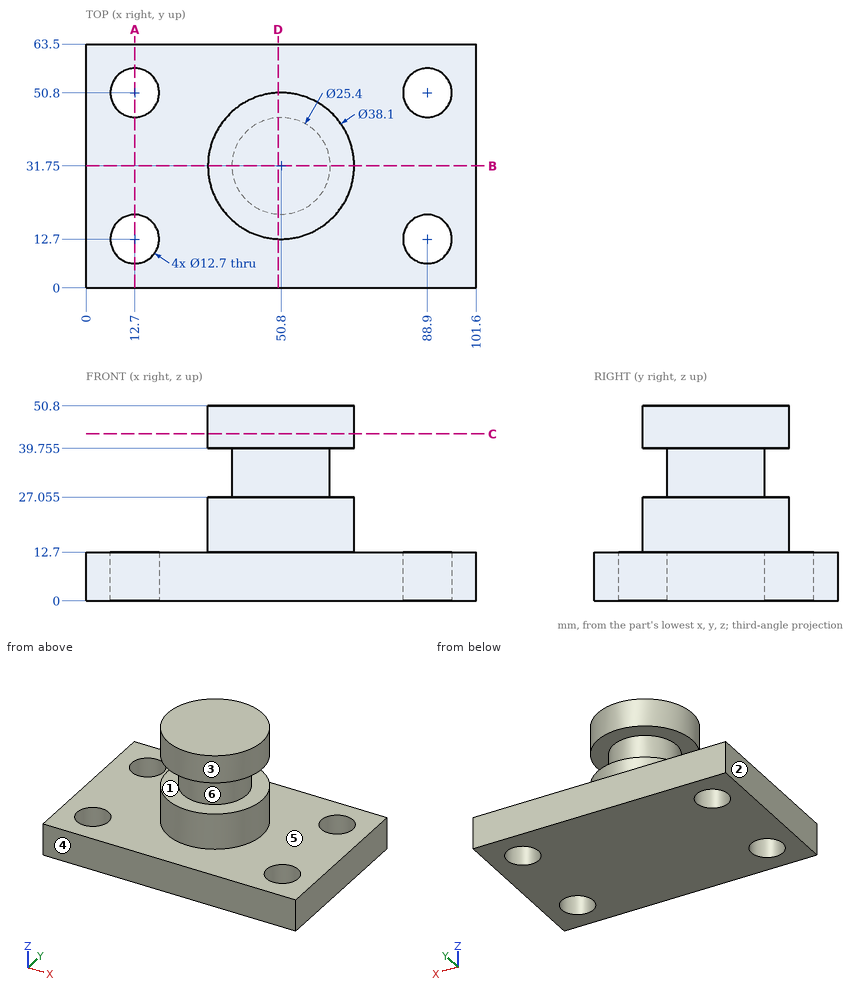
For this review, use the dimensioned drawing (mm, ordinates from the lowest corner) and the shaded views. A direction names the side the tool comes from. Coordinates: 2 decimals unless noted, no trailing zeros. Write each loop counter-clockwise with the first axis right and the second up, starting at its lowest first coordinate (ties: lowest second). Pieces come first, ordered by that corner, then holes. Notation, with made-up numbers: (65, 43) -> (83, 43) arc R25 cw to (83, 80) -> close; hole circle Ø2 at (28.5, 8). An arc over 180 degrees is marked (long way). Put each result on its own line as item: value.
Q1. Take a section at A-A, the plane x = 12.7. State the section outline as (y, z) points, then the cut area to 3 significant figures.
From the geometry:
outline: (0, 0) -> (6.35, 0) -> (6.35, 12.7) -> (0, 12.7) -> close; (19.05, 0) -> (44.45, 0) -> (44.45, 12.7) -> (19.05, 12.7) -> close; (57.15, 0) -> (63.5, 0) -> (63.5, 12.7) -> (57.15, 12.7) -> close
area: 484 mm2
Q2. Take a section at D-D, the plane x = 50. State the section outline as (y, z) points (1 decimal), then the cut area to 3 significant figures.
From the geometry:
outline: (0, 0) -> (63.5, 0) -> (63.5, 12.7) -> (50.8, 12.7) -> (50.8, 27.1) -> (44.4, 27.1) -> (44.4, 39.8) -> (50.8, 39.8) -> (50.8, 50.8) -> (12.7, 50.8) -> (12.7, 39.8) -> (19.1, 39.8) -> (19.1, 27.1) -> (12.7, 27.1) -> (12.7, 12.7) -> (0, 12.7) -> close
area: 2,100 mm2
Q3. The part is to be moulded in two halves that separate along Z. For the marked faces 4, 5 and 6, say which applies: +Z half, -Z half, draft (parallel to the pull), parting line (faces both ways), or undercut.
From the geometry:
face 4: draft
face 5: +Z half
face 6: undercut
Q4. Clearance check with flat-ended pins moving along their axes: pin 1 Ø11.5 at (x, y) = (88.9, 50.8) entering from -Z; pin 2 Ø8 at (x, y) = (59, 54.5) entering from +Z; pin 3 Ø2 at (x, y) = (30, 27.5) entering from -Z; pin 4 Ø8 at (x, z) = (38.5, 39) entering from -Y. State where each tip first meets the part, or that it passes through.
From the geometry:
pin 1: passes through
pin 2: stops at z = 12.7
pin 3: stops at z = 0
pin 4: stops at y = 14.64
Q5. Wall thickness on L1, parallel to Y at x = 88.9, z = 6.75; L2, parallel to X at y = 50, z = 9; L3, parallel to Y at x = 14, z = 7: over which ranges is each line inside the solid? List them lowest first.
From the geometry:
L1: y = 0 to 6.35, 19.05 to 44.45, 57.15 to 63.5
L2: x = 0 to 6.4, 19 to 82.6, 95.2 to 101.6
L3: y = 0 to 6.48, 18.92 to 44.58, 57.02 to 63.5
Q6. Tool access review of the marked faces 1, 2 and 3: name each direction out of +Z, -Z, +X, -X, +Y, -Y from which nothing blocks a thin tool from reaching the whole face with its end or side.
From the geometry:
face 1: none
face 2: +Z, -Z, -X, +Y, -Y
face 3: +Z
Q7. Take a section at C-C, the plane z = 43.5. State the section outline as (x, y) points, then the cut area to 3 significant figures.
From the geometry:
outline: circle Ø38.1 at (50.8, 31.75)
area: 1,140 mm2
Q8. Take a section at B-B, the plane y = 31.75. State the section outline as (x, z) points (3 decimals).
From the geometry:
outline: (0, 0) -> (101.6, 0) -> (101.6, 12.7) -> (69.85, 12.7) -> (69.85, 27.055) -> (63.5, 27.055) -> (63.5, 39.755) -> (69.85, 39.755) -> (69.85, 50.8) -> (31.75, 50.8) -> (31.75, 39.755) -> (38.1, 39.755) -> (38.1, 27.055) -> (31.75, 27.055) -> (31.75, 12.7) -> (0, 12.7) -> close
